```python
from build123d import *

# Parameters (mm, degrees)
SKETCH1_R                             = 30
ARCH_OUTER_DEPTH                      = 3
WHEEL_CLEARANCE_R27_START             = -0.1
SKETCH2_R                             = 27
WHEEL_CLEARANCE_R27_DEPTH             = 3.2
OPEN_BOTTOM_AT_GROUND_CLEARANCE_START = -0.1
SKETCH3_W                             = 62
SKETCH3_H                             = 20.5
OPEN_BOTTOM_AT_GROUND_CLEARANCE_DEPTH = 3.2


with BuildPart() as part:
    # Sketch1 → Arch_Outer (new body)
    with BuildSketch(Plane.XY):
        Circle(SKETCH1_R)
    extrude(amount=ARCH_OUTER_DEPTH)

    # Sketch2 → Wheel_Clearance_R27 (cut)
    with BuildSketch(Plane.XY.offset(WHEEL_CLEARANCE_R27_START)):
        Circle(SKETCH2_R)
    extrude(amount=WHEEL_CLEARANCE_R27_DEPTH, mode=Mode.SUBTRACT)

    # Sketch3 → Open_Bottom_At_Ground_Clearance (cut)
    with BuildSketch(Plane.XY.offset(OPEN_BOTTOM_AT_GROUND_CLEARANCE_START)):
        with Locations((0, -20.75)):
            Rectangle(SKETCH3_W, SKETCH3_H)
    extrude(amount=OPEN_BOTTOM_AT_GROUND_CLEARANCE_DEPTH, mode=Mode.SUBTRACT)


solid = part.part
```
Work out the finished part from the listing and answer in its coordinate system (mm). Give positions to 0.01 mm unless a question says otherwise; leave off trailing zeros. Loops run counter-clockwise (first coordinate to the right, second up) from the corner with the lowest first, then second, coordinate; pieces in that order, holes last. Notation, with made-up numbers: (5, 32.5) -> (14, 32.5) arc R18 cw to (14, 65.5) -> close; hole circle Ø8 at (82, 75.5). An arc over 180 degrees is marked (long way). One line per question, with ' | ' between items. Start each with the question number.
1) Section C-C, the plane y = 20 is taken. Determine the outline of the cut face in (x, z).
2) Section D-D, the plane z = 0.8 is taken. Determine the outline of the cut face in (x, y).
3) Section B-B, the plane x = 0 is taken. Determine the outline of the cut face in (y, z), then the cut area to 3 significant figures.
4) This flat-tipped pin is pushed along its axis until it touches: pin 1 (1.5 mm diameter, centred on x = 8.5, z = 0.5, fed in from -Y). Where does it stop, or does it pass through?
5) Section A-A, the plane y = 0 is taken. Determine the outline of the cut face in (x, z), then the cut area to 3 significant figures.
6) Determine the mould class of faces 1 (the face through (0.74, 26.99, 1.48)), 2 (the face through (0.81, 29.99, 1.48)), 3 (the face through (-27, -10.5, 1)) for opening direction Y: +Y half, -Y half, draft (parallel to the pull), parting line (faces both ways), or undercut.
7) Straight lines are drawn through the part: L1, parallel to X at y = 0, z = 1.6; L2, parallel to Y at x = 0, z = 1.6; L3, parallel to X at y = 5, z = 2.05. For each, find the intervals that lie inside material, in ascending order.
Resolved:
1) outline: (-22.36, 0) -> (-18.14, 0) -> (-18.14, 3) -> (-22.36, 3) -> close; (18.14, 0) -> (22.36, 0) -> (22.36, 3) -> (18.14, 3) -> close
2) outline: (-28.1, -10.5) -> (-24.87, -10.5) arc R27 cw (long way) to (24.87, -10.5) -> (28.1, -10.5) arc R30 ccw (long way) to start
3) outline: (27, 0) -> (30, 0) -> (30, 3) -> (27, 3) -> close | area: 9.00 mm2
4) pin 1: y = 25.37
5) outline: (-30, 0) -> (-27, 0) -> (-27, 3) -> (-30, 3) -> close; (27, 0) -> (30, 0) -> (30, 3) -> (27, 3) -> close | area: 18.0 mm2
6) face 1: undercut | face 2: parting line | face 3: -Y half
7) L1: -30 to -27, 27 to 30 | L2: 27 to 30 | L3: -29.58 to -26.53, 26.53 to 29.58
